```python
from build123d import *

# Parameters (mm, degrees)
SKETCH1_W           = 194
SKETCH1_H           = 100
BOSS_EXTRUDE1_DEPTH = 1
SKETCH2_R           = 1.75
BOSS_EXTRUDE2_DEPTH = 1
SKETCH5_W           = 8
SKETCH5_H           = 108
BOSS_EXTRUDE3_DEPTH = 1
CUT_EXTRUDE3_DEPTH  = 219.249856816


with BuildPart() as part:
    # Sketch1 → Boss-Extrude1 (new body)
    with BuildSketch(Plane(origin=(0, 0, 0), x_dir=(1, 0, 0), z_dir=(0, 1, 0))):
        Rectangle(SKETCH1_W, SKETCH1_H)
    extrude(amount=BOSS_EXTRUDE1_DEPTH)

    # Sketch2 → Boss-Extrude2 (add)
    with BuildSketch(Plane.ZY.offset(97)):
        with BuildLine():
            Line((58, 0), (58, 9))
            ThreePointArc((58, 9), (54, 13), (50, 9))
            Line((50, 9), (50, 0))
            Line((50, 0), (58, 0))
        make_face()
        with Locations((54, 9)):
            Circle(SKETCH2_R, mode=Mode.SUBTRACT)
    boss_extrude2 = extrude(amount=-BOSS_EXTRUDE2_DEPTH)

    # Mirror1: Boss-Extrude2 across plane
    add(boss_extrude2.mirror(Plane.ZY))

    # Sketch5 → Boss-Extrude3 (add)
    with BuildSketch(Plane(origin=(0, 1, 0), x_dir=(1, 0, 0), z_dir=(0, 1, 0))):
        with Locations((-101, -4)):
            Rectangle(SKETCH5_W, SKETCH5_H)
        with Locations((101, -4)):
            Rectangle(SKETCH5_W, SKETCH5_H)
    extrude(amount=-BOSS_EXTRUDE3_DEPTH)

    # Sketch6 → Cut-Extrude3 (cut, through all)
    with BuildSketch(Plane.ZY.offset(105)):
        with BuildLine():
            Line((58, 0), (56, 0))
            ThreePointArc((56, 0), (57.414213562, 0.585786438), (58, 2))
            Line((58, 2), (58, 0))
        make_face()
    extrude(amount=-CUT_EXTRUDE3_DEPTH, mode=Mode.SUBTRACT)


solid = part.part
```
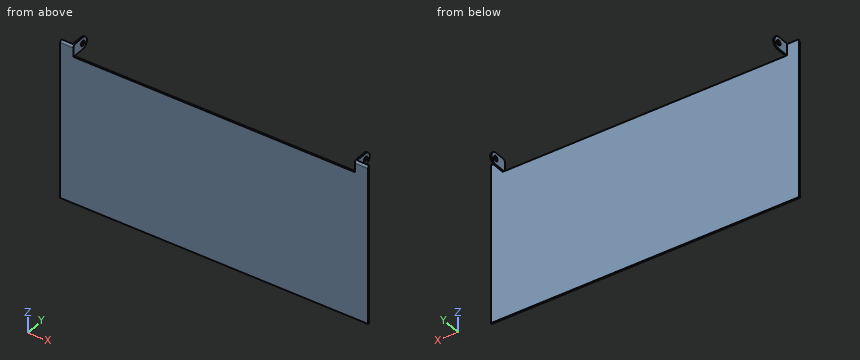
Verification items for the finished model (mm, model axes). Round coordinates to 2 decimals unless told otherwise and drop trailing zeros. Order: outer loops, then holes, each group sorted by start corner. A loop starts at its lowest first (then second) coordinate and runs counter-clockwise, first axis right, second up. Notation, with made-up numbers: (-26.75, -35.5) - (-1.75, -35.5) arc R19 cw to (-1.75, -24.5) - close; hole circle Ø1 at (41.5, -38.75). An arc over 180 degrees is marked (long way). Use CSV: the item, a comma, the result in double quotes.
(1) Section check A-A on z = 16.5. Record the boundary of the cut face in (x, y).
Entries:
outline,"(-105, 0) - (105, 0) - (105, 1) - (-105, 1) - close"
(2) Thickness scan on probe 1 along X at (y, z) = (10, 51.5); probe 2 along Y at (x, z) = (-96.4, 54); probe 3 along Z at (x, y) = (-32.5, 0.5). Record the ranges inside material, lowest first. Write a range as from..to.
Entries:
probe 1,"-97..-96, 96..97"
probe 2,"0..7.25, 10.75..13"
probe 3,"-50..50"
(3) Gauge pin test, flat ends, axial feed: pin 1 Ø5.5 at (y, z) = (9, 54) entering from +X; pin 2 Ø3 at (y, z) = (9, 54) entering from +X; pin 3 Ø6 at (x, z) = (47, 17.5) entering from +Y; pin 4 Ø0.5 at (x, y) = (96.5, 6) entering from -Z. Record the tip position at first contact, or that the pin passes through.
Entries:
pin 1,"x = 97"
pin 2,"through"
pin 3,"y = 1"
pin 4,"z = 50"
(4) Section check B-B on x = -63.5. Record the boundary of the cut face in (y, z).
Entries:
outline,"(0, -50) - (1, -50) - (1, 50) - (0, 50) - close"
